Verification items for this drawing (mm, ordinates from the low corner). Coordinates: 2 decimals unless noted, no trailing zeros. Write each loop counter-clockwise with the first axis right and the second up, starting at its lowest first coordinate (ties: lowest second). Pieces come first, ordered by that corner, then holes. Notation, with made-up numbers: M 87,-20.5 L 138,-20.5 A19 cw 138,16.5 Z; hole C 59,-23 d9. An arc over 180 degrees is marked long. Put each result on its own line as item: value. Start each with the question number.
1) Cross-section at A-A on x = 5. Record the cut outline in (y, z).
2) Cross-section at C-C on z = 1.65. Record the cut outline in (x, y).
3) Scan line: line 1 along Y through (x, z) = (5, 1.7). Record every from-to range of solid material in increasing order.
4) Cross-section at B-B on y = 35. Record the cut outline in (x, z), plus the area to 3 significant figures.
5) Mould release check, pull along X, two halves, no side actions. Record for the marked faces 1, 2 and 3: released by +X, released by -X, zero draft, split by the parting line, or undercut.
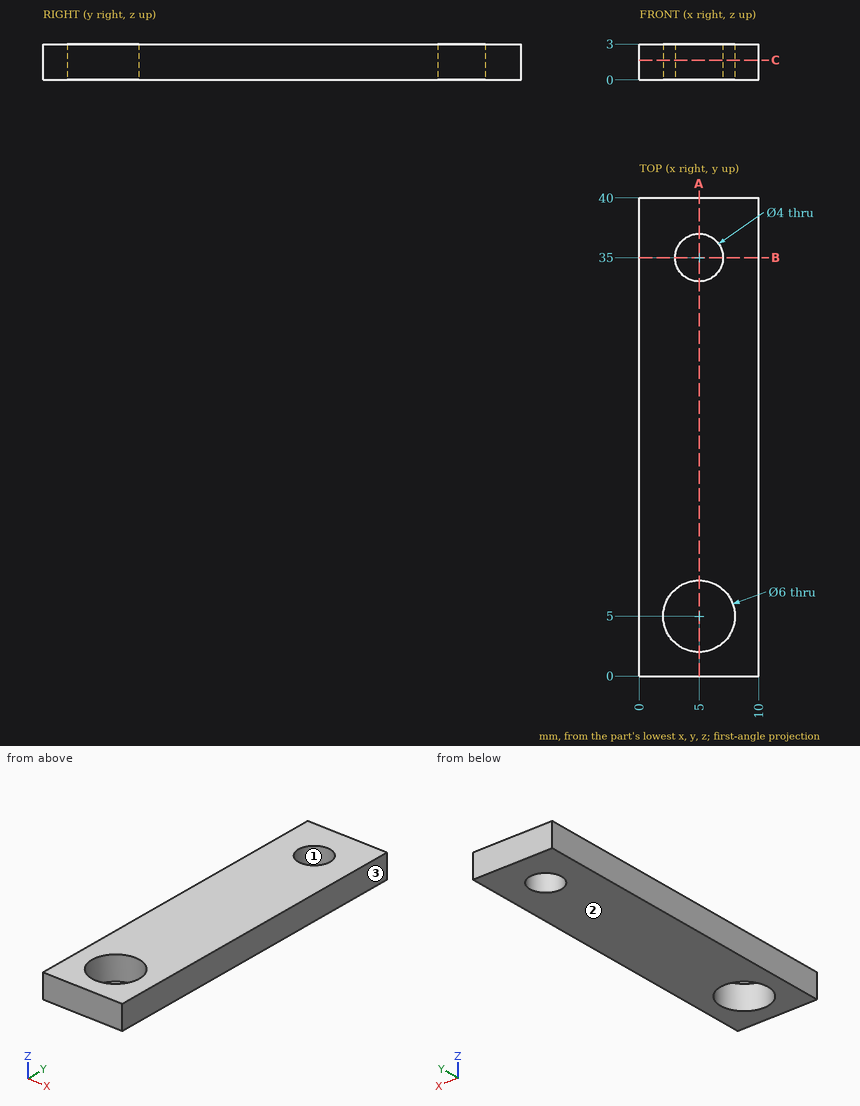
Answer key:
1. outline: M 0,0 L 2,0 L 2,3 L 0,3 Z; M 8,0 L 33,0 L 33,3 L 8,3 Z; M 37,0 L 40,0 L 40,3 L 37,3 Z
2. outline: M 0,0 L 10,0 L 10,40 L 0,40 Z; hole C 5,5 d6; hole C 5,35 d4
3. line 1: y = 0 to 2, 8 to 33, 37 to 40
4. outline: M 0,0 L 3,0 L 3,3 L 0,3 Z; M 7,0 L 10,0 L 10,3 L 7,3 Z
4. area: 18.0 mm²
5. face 1: undercut
5. face 2: zero draft
5. face 3: released by +X
